Source: CAD feature listing. Evaluate the final solid. Frame: model axes, mm. Face numbers are marked on the shaded views. A direction names the side the tool comes from. Give positions to 0.01 mm unless a question says otherwise; leave off trailing zeros. Write each loop counter-clockwise with the first axis right and the second up, starting at its lowest first coordinate (ties: lowest second). Pieces come first, ordered by that corner, then holes. Notation, with made-up numbers: (31, 77) - (71, 77) arc R10 ccw to (71, 83) - close; hole circle Ø7 at (21, 38). An arc over 180 degrees is marked (long way). One line per question, with ' | ' between items. Start each with the question number.
(1) Pin query (flat end, axial travel): pin 1 (2 mm diameter, centred on y = -37, z = 23, fed in from +X); pin 2 (5 mm diameter, centred on y = -67.5, z = 0, fed in from +X); pin 3 (1 mm diameter, centred on y = -49, z = -19.5, fed in from -X). Return the tip coordinate at first contact, or that it passes through.
(2) Section C-C, the plane y = -121.5. Return loops of the section in (x, z), plus the area to 3 significant figures.
(3) Ray query, line 1 (Y direction, x = 24, z = 53); line 2 (Z direction, x = -33, y = -52); line 3 (X direction, y = -113.5, z = -6). Return the intervals inside material, ascending. Write a range as [from, to].
(4) Section B-B, the plane x = -17. Return loops of the section in (y, z), plus the area to 3 significant figures.
(5) Access query for the marked faces 4, 5 and 6. Directions: +Z, -Z, +X, -X, +Y, -Y. A direction counts if a zero-diameter tool reaches every point of the face in a straight line with its end or side. Return the directions, or none.
(6) Section D-D, the plane z = 41.5. Return loops of the section in (x, y).
(7) Section A-A, the plane z = -43. Return loops of the section in (x, y), plus the area to 3 significant figures.
(8) Draft query along X for the marked faces 1, 2 and 3. Return one class per face: +X half, -X half, draft (parallel to the pull), parting line (faces both ways), or undercut.
```python
from build123d import *

# Parameters (mm, degrees)
F0_W          = 145.2813223004
F0_H          = 106.4100638032
F1_DEPTH      = 152.4
F3_DEPTH      = 25.4
F3_DEPTH_BACK = 193.04
F4_R          = 14.1433096913
F5_DEPTH      = 41.402
F7_DEPTH      = 25.4


with BuildPart() as f1:
    # F0 (on Front) → F1 (new body)
    with BuildSketch(Plane.XZ):
        with Locations((14.9816311896, -2.8343647718)):
            Rectangle(F0_W, F0_H)
    extrude(amount=F1_DEPTH)

    # F2 (on Front) → F3 (cut, two sides)
    with BuildSketch(Plane.XZ) as f3_sk:
        Polygon((91.3226157427, 59.4377643871), (0, 58.912049979), (91.3226157427, -60.7426390052), align=None)
    extrude(amount=-F3_DEPTH, mode=Mode.SUBTRACT)
    extrude(f3_sk.sketch, amount=F3_DEPTH_BACK, mode=Mode.SUBTRACT)

    # F4 (on face) → F5 (cut)
    with BuildSketch(Plane(origin=(28.4124414854, 0, 21.6848875552), x_dir=(0, 1, 0), z_dir=(0.794928192, 0, 0.6067035269))):
        with Locations((-74.8865753412, -20.3293599188)):
            Circle(F4_R)
    extrude(amount=-F5_DEPTH, mode=Mode.SUBTRACT)

    # F6 (on Front) → F7 (join)
    with BuildSketch(Plane.XZ):
        Polygon((9.9221970886, 76.122879982), (-57.940531522, 76.122879982), (-57.940531522, -56.0393966734), (99.3260890245, -56.0393966734), (99.3260890245, -34.1743119061), align=None)
    extrude(amount=F7_DEPTH)


solid = f1.part
```
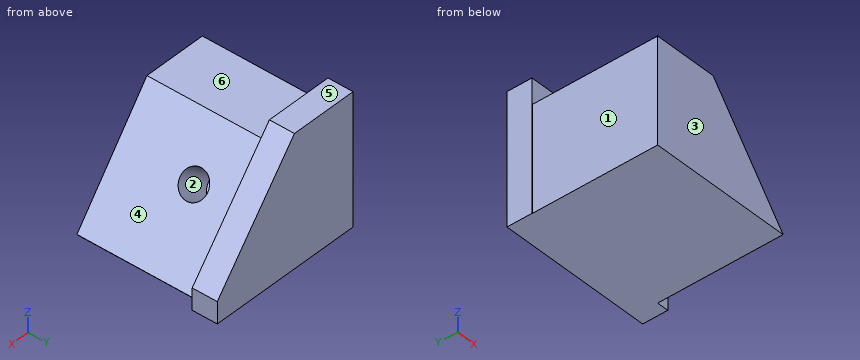
Check sheet entries:
1) pin 1: x = 28.17 | pin 2: x = 18.06 | pin 3: x = -57.66
2) outline: (-57.66, -56.04) - (87.62, -56.04) - (87.62, -55.89) - (6.52, 50.37) - (-57.66, 50.37) - close | area: 11,200 mm²
3) line 1: [-25.4, 0] | line 2: [-56.04, 50.37] | line 3: [-57.66, 49.54]
4) outline: (-152.4, -56.04) - (0, -56.04) - (0, 76.12) - (-25.4, 76.12) - (-25.4, 50.37) - (-152.4, 50.37) - close | area: 16,900 mm²
5) face 4: +Z, +X, -Y | face 5: +Z, +X, -X, +Y, -Y | face 6: +Z, +X, -X, -Y
6) outline: (-57.94, -25.4) - (-57.66, -25.4) - (-57.66, -152.4) - (13.29, -152.4) - (13.29, -25.4) - (37.99, -25.4) - (37.99, 0) - (-57.94, 0) - close
7) outline: (-57.94, -25.4) - (-57.66, -25.4) - (-57.66, -152.4) - (77.78, -152.4) - (77.78, -25.4) - (99.33, -25.4) - (99.33, 0) - (-57.94, 0) - close | area: 21,200 mm²
8) face 1: -X half | face 2: undercut | face 3: draft
